from build123d import *

# Parameters (mm, degrees)
SKETCH_1_W          = 29
SKETCH_1_H          = 65
EXTRUDE_1_DEPTH     = 25
SKETCH_2_R          = 3.025
SKETCH_2_R_2        = 3.005
CUT_EXTRUDE_3_DEPTH = 76.43871685
SKETCH_6_W          = 14.5
SKETCH_6_H          = 65
CUT_EXTRUDE_4_DEPTH = 76.43871685
SKETCH_7_R          = 2
CUT_EXTRUDE_5_DEPTH = 72.135434208
SKETCH_8_R          = 2
CUT_EXTRUDE_6_DEPTH = 72.135434208
SKETCH_9_R          = 2
CUT_EXTRUDE_7_DEPTH = 72.135434208


with BuildPart() as part:
    # 草图1 → 凸台-拉伸1 (new body)
    with BuildSketch(Plane.XY):
        with Locations((14.5, 32.5)):
            Rectangle(SKETCH_1_W, SKETCH_1_H)
    extrude(amount=EXTRUDE_1_DEPTH)

    # 草图2 → 切除-拉伸3 (cut, through all)
    # profile 1 of 2: a face of its own
    with BuildSketch(Plane.XY.offset(25)):
        with Locations((14.5, 52)):
            Circle(SKETCH_2_R)
        with Locations((14.5, 52)):
            Circle(SKETCH_2_R_2, mode=Mode.SUBTRACT)
    # profile 2 of 2: a face of its own
    with BuildSketch(Plane.XY.offset(25)):
        with Locations((14.5, 18)):
            Circle(SKETCH_2_R)
        with Locations((14.5, 18)):
            Circle(SKETCH_2_R_2, mode=Mode.SUBTRACT)
    extrude(amount=-CUT_EXTRUDE_3_DEPTH, mode=Mode.SUBTRACT)


with BuildPart() as cut_extrude_3_kept_piece:
    # of the separate pieces the step leaves, the one the design keeps (cut_extrude_3_pieces_kept)
    add(part.part.solids().sort_by_distance((0, 0, 0))[0])

    # 草图6 → 切除-拉伸4 (cut, through all)
    with BuildSketch(Plane.XY.offset(25)):
        with Locations((21.75, 32.5)):
            Rectangle(SKETCH_6_W, SKETCH_6_H)
    extrude(amount=-CUT_EXTRUDE_4_DEPTH, mode=Mode.SUBTRACT)

    # 草图7 → 切除-拉伸5 (cut, through all)
    with BuildSketch(Plane(origin=(14.5, 0, 0), x_dir=(0, 0, -1), z_dir=(1, 0, 0))):
        with Locations((-20, 60.0125)):
            Circle(SKETCH_7_R)
        with Locations((-5, 60.0125)):
            Circle(SKETCH_7_R)
    extrude(amount=-CUT_EXTRUDE_5_DEPTH, mode=Mode.SUBTRACT)

    # 草图8 → 切除-拉伸6 (cut, through all)
    with BuildSketch(Plane(origin=(14.5, 0, 0), x_dir=(0, 0, -1), z_dir=(1, 0, 0))):
        with Locations((-20, 35)):
            Circle(SKETCH_8_R)
        with Locations((-5, 35)):
            Circle(SKETCH_8_R)
    extrude(amount=-CUT_EXTRUDE_6_DEPTH, mode=Mode.SUBTRACT)

    # 草图9 → 切除-拉伸7 (cut, through all)
    with BuildSketch(Plane(origin=(14.5, 0, 0), x_dir=(0, 0, -1), z_dir=(1, 0, 0))):
        with Locations((-20, 7.4875)):
            Circle(SKETCH_9_R)
        with Locations((-5, 7.4875)):
            Circle(SKETCH_9_R)
    extrude(amount=-CUT_EXTRUDE_7_DEPTH, mode=Mode.SUBTRACT)


solid = cut_extrude_3_kept_piece.part
CAD build for the part. Positions are in the model's coordinates, mm. Round coordinates to 2 decimals unless told otherwise and drop trailing zeros. Write each loop counter-clockwise with the first axis right and the second up, starting at its lowest first coordinate (ties: lowest second). Pieces come first, ordered by that corner, then holes. Notation, with made-up numbers: M 41.25,-14 L 48.25,-14 A21 cw 48.25,23 Z; hole C -6.5,16 d5. An arc over 180 degrees is marked long. Put each result on its own line as item: value. Start each with the question number.
1) Saw through at D-D, the plane z = 10.75. Write the cut outline in (x, y) (3 decimals).
2) Pin check, flat tip, straight feed: pin 1 Ø5 at (y, z) = (46.5, 21.5) entering from -X. Stop position of the tip, or through.
3) Pull direction Y, two halves, no side cores. Call faces 1 (the cylindrical face through (7, 33, 5)), 2 (the cylindrical face through (11.476, 18.067, 12.675)), 3 (the flat face through (7, 33, 25)), 4 (the flat face through (7, 65, 12)): pulls with the +Y half, pulls with the -Y half, needs draft (parallel to the pull), parting line crosses it, or undercut.
4) Saw through at B-B, the plane y = 35. Write the cut outline in (x, z), and give its area (4 significant figures).
5) Drill centre lines: probe 1 along Y at (x, z) = (9.75, 5); probe 2 along Y at (x, z) = (13.25, 4.5); probe 3 along Z at (x, y) = (11, 35.5). Where is each one in solid material? Low to high. Write a range as [from, to].
6) Saw through at A-A, the plane z = 20. Count the separate pieces of the cut face and the enclosed holes in it, and give its area (3 significant figures).
Resolved:
1. outline: M 0,0 L 14.5,0 L 14.5,14.975 A3.025 cw 14.5,21.025 L 14.5,48.975 A3.025 cw 14.5,55.025 L 14.5,65 L 0,65 Z
2. pin 1: x = 0
3. face 1: undercut
3. face 2: undercut
3. face 3: needs draft
3. face 4: pulls with the +Y half
4. outline: M 0,0 L 14.5,0 L 14.5,3 L 0,3 Z; M 0,7 L 14.5,7 L 14.5,18 L 0,18 Z; M 0,22 L 14.5,22 L 14.5,25 L 0,25 Z
4. area: 246.5 mm²
5. probe 1: [0, 5.49], [9.49, 33], [37, 58.01], [62.01, 65]
5. probe 2: [0, 5.55], [9.42, 15.25], [20.75, 33.06], [36.94, 49.25], [54.75, 58.08], [61.95, 65]
5. probe 3: [0, 3.06], [6.94, 18.06], [21.94, 25]
6. separate pieces: 4
6. enclosed holes: 0
6. area: 740 mm²
